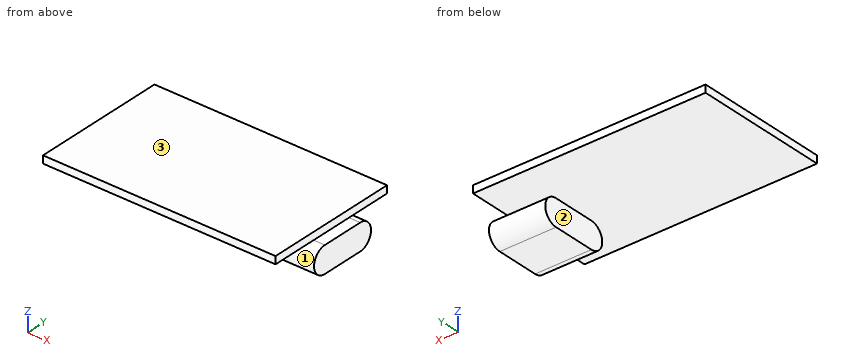
from build123d import *

# Parameters (mm, degrees)
ESBO_O1_W                     = 31
ESBO_O1_H                     = 18
RESSALTO_EXTRUS_O1_DEPTH      = 1
RESSALTO_EXTRUS_O2_DEPTH      = 1.5
RESSALTO_EXTRUS_O2_DEPTH_BACK = 6


with BuildPart() as part:
    # Esboço1 → Ressalto-extrusão1 (new body)
    with BuildSketch(Plane.XY):
        Rectangle(ESBO_O1_W, ESBO_O1_H)
    extrude(amount=RESSALTO_EXTRUS_O1_DEPTH)

    # Esboço2 → Ressalto-extrusão2 (add, two sides)
    with BuildSketch(Plane(origin=(15.5, 0, 0), x_dir=(0, 0, -1), z_dir=(1, 0, 0))) as ressalto_extrus_o2_sk:
        with BuildLine():
            Line((3.5, 2.85), (3.5, -2.85))
            ThreePointArc((3.5, -2.85), (1.75, -4.6), (0, -2.85))
            Line((0, -2.85), (0, 2.85))
            ThreePointArc((0, 2.85), (1.75, 4.6), (3.5, 2.85))
        make_face()
    extrude(amount=RESSALTO_EXTRUS_O2_DEPTH)
    extrude(ressalto_extrus_o2_sk.sketch, amount=-RESSALTO_EXTRUS_O2_DEPTH_BACK)


solid = part.part
Input: part model. Units: mm. Frame: model coordinates. Face numbers are marked on the shaded views. Give positions to 0.01 mm unless a question says otherwise; leave off trailing zeros. Order: outer loops, then holes, each group sorted by start corner. A loop starts at its lowest first (then second) coordinate and runs counter-clockwise, first axis right, second up. Notation, with made-up numbers: M 24.5,47.5 L 30.5,47.5 A16 ccw 30.5,60.5 Z; hole C -36,13.5 d9. An arc over 180 degrees is marked long. Answer as a JSON object with one key per item and string values.
1. Ray query, line 1 (Z direction, x = -11, y = -7.5); line 2 (X direction, y = 6.5, z = 0.05); line 3 (X direction, y = -1.25, z = -1.6). Return the intervals inside material, ascending. Write a range as [from, to].
Result sheet:
{"line 1": "[0, 1]", "line 2": "[-15.5, 15.5]", "line 3": "[9.5, 17]"}
2. First-contact query: P1, Ø5.5, axis at x = -2.5, y = 0, coming from the -Z side; P2, Ø1, axis at y = 0, z = -2.5, coming from the -X side; P3, Ø1.6, axis at x = 16, y = 0.5, coming from the +Z side. Flat tips, straight axial feed; report the tip coordinate or a pass-through.
Result sheet:
{"P1": "z = 0", "P2": "x = 9.5", "P3": "z = 1"}
3. Cut plane A-A, the plane x = 12.5. Output: boundary loops of the cut face in (y, z), and give its area (3 significant figures).
Result sheet:
{"outline": "M -9,0 L -2.85,0 A1.75 ccw -2.85,-3.5 L 2.85,-3.5 A1.75 ccw 2.85,0 L 9,0 L 9,1 L -9,1 Z", "area": "47.6 mm²"}
4. Cut plane C-C, the plane z = -0.7. Output: boundary loops of the cut face in (x, y).
Result sheet:
{"outline": "M 9.5,-4.25 L 17,-4.25 L 17,4.25 L 9.5,4.25 Z"}
5. Cut plane D-D, the plane x = -6. Output: boundary loops of the cut face in (y, z).
Result sheet:
{"outline": "M -9,0 L 9,0 L 9,1 L -9,1 Z"}
6. Pull-direction query (Z, two-part tool) for the marked faces 1, 2 and 3; classes: +Z half, -Z half, draft (parallel to the pull), parting line (faces both ways), or undercut.
Result sheet:
{"face 1": "undercut", "face 2": "draft", "face 3": "+Z half"}
7. Cut plane B-B, the plane y = 2. Output: boundary loops of the cut face in (x, z).
Result sheet:
{"outline": "M -15.5,0 L 9.5,0 L 9.5,-3.5 L 17,-3.5 L 17,0 L 15.5,0 L 15.5,1 L -15.5,1 Z"}
